```python
from build123d import *

# Parameters (mm, degrees)
SKETCH1_R           = 7.14375
BOSS_EXTRUDE1_DEPTH = 10.25
SKETCH2_R           = 11.75
BOSS_EXTRUDE2_DEPTH = 25
SKETCH6_R           = 4
CUT_EXTRUDE4_DEPTH  = 20
CUT_EXTRUDE5_START  = -20
CUT_EXTRUDE5_DEPTH  = 20
SKETCH7_R           = 4
CUT_EXTRUDE6_DEPTH  = 30
FILLET1_R           = 2.5
FILLET2_R           = 2.5


with BuildPart() as part:
    # Sketch1 → Boss-Extrude1 (new body)
    with BuildSketch(Plane(origin=(0, 0, 0), x_dir=(1, 0, 0), z_dir=(0, 1, 0))):
        with Locations(Location((0, 0, 0), (0, 0, 270))):
            Circle(SKETCH1_R)
    extrude(amount=BOSS_EXTRUDE1_DEPTH)

    # Sketch2 → Boss-Extrude2 (add)
    with BuildSketch(Plane(origin=(0, 10.25, 0), x_dir=(1, 0, 0), z_dir=(0, 1, 0))):
        with Locations(Location((0, 0, 0), (0, 0, 270))):
            Circle(SKETCH2_R)
    extrude(amount=BOSS_EXTRUDE2_DEPTH)

    # Sketch6 → Cut-Extrude4 (cut)
    with BuildSketch(Plane.XZ):
        with Locations(Location((0, 0, 0), (0, 0, 270))):
            Circle(SKETCH6_R)
    extrude(amount=-CUT_EXTRUDE4_DEPTH, mode=Mode.SUBTRACT)

    # Sketch3 → Cut-Extrude5 (cut)
    with BuildSketch(Plane(origin=(0, 35.25, 0), x_dir=(1, 0, 0), z_dir=(0, 1, 0)).offset(CUT_EXTRUDE5_START)):
        with BuildLine():
            ThreePointArc((6.05, 10.072735478), (0, 11.75), (-6.05, 10.072735478))
            Line((-6.05, 10.072735478), (-6.05, -10.072735478))
            ThreePointArc((-6.05, -10.072735478), (0, -11.75), (6.05, -10.072735478))
            Line((6.05, -10.072735478), (6.05, 10.072735478))
        make_face()
        with BuildLine():
            Line((-10.25, -5.744562647), (-10.25, 5.744562647))
            ThreePointArc((-10.25, 5.744562647), (-11.75, 0), (-10.25, -5.744562647))
        make_face()
        with BuildLine():
            ThreePointArc((11.75, 0), (11.368817001, 2.968585522), (10.25, 5.744562647))
            Line((10.25, 5.744562647), (10.25, -5.744562647))
            ThreePointArc((10.25, -5.744562647), (11.368817001, -2.968585522), (11.75, 0))
        make_face()
    extrude(amount=CUT_EXTRUDE5_DEPTH, mode=Mode.SUBTRACT)

    # Sketch7 → Cut-Extrude6 (cut)
    with BuildSketch(Plane.ZY.offset(10.25)):
        with Locations((0, 26.25)):
            Circle(SKETCH7_R)
    extrude(amount=-CUT_EXTRUDE6_DEPTH, mode=Mode.SUBTRACT)

    # Fillet1
    fillet1_edges = [part.edges().sort_by_distance(p)[0] for p in [
        (10.25, 25.25, -5.744562647),
        (10.25, 25.25, 5.744562647),
        (-10.25, 25.25, -5.744562647),
        (-10.25, 25.25, 5.744562647),
    ]]
    fillet(fillet1_edges, radius=FILLET1_R)

    # Fillet2
    fillet2_edges = [part.edges().sort_by_distance(p)[0] for p in [
        (-8.155066755, 35.25, -8.4591599),
        (8.155066755, 35.25, 8.4591599),
        (8.155066755, 35.25, -8.4591599),
        (-8.155066755, 35.25, 8.4591599),
        (10.25, 35.25, 0),
        (10.146506466, 35.25, -5.761620966),
        (10.146506466, 35.25, 5.761620966),
        (-10.25, 35.25, 0),
        (-10.146506466, 35.25, -5.761620966),
        (-10.146506466, 35.25, 5.761620966),
    ]]
    fillet(fillet2_edges, radius=FILLET2_R)


solid = part.part
```
Can you work these out from the model? Positions are in its coordinate system, mm. A direction names the side the tool comes from. Coordinates: 2 decimals unless noted, no trailing zeros. Write each loop counter-clockwise with the first axis right and the second up, starting at its lowest first coordinate (ties: lowest second). Pieces come first, ordered by that corner, then holes. Notation, with made-up numbers: M 3,-36 L 62,-36 A29 cw 62,-13 Z; hole C 30.25,23.5 d4. An arc over 180 degrees is marked long. Write item = value, one per line. Start each with the question number.
Q1. If we section it at D-D, the plane y = 20.5: Write out the boundary of the cut face in (x, z), then the cut area to 3 significant figures.
Q2. If we section it at C-C, the plane z = 0: State how many separate pieces and enclosed holes the cut face has, then the cut area to 3 significant figures.
Q3. I'm going to push flat-ended pins straight in: pin 1 (1 mm diameter, centred on x = 10.5, z = 0, fed in from +Y); pin 2 (5 mm diameter, centred on y = 20.5, z = 0, fed in from -X); pin 3 (10 mm diameter, centred on y = 30, z = 3.5, fed in from +X). Where does each tip first touch, or does it pass through?
Q4. Thinking about a two-plate mould opening in Y: for faces 6 (the face through (-8.179, 30.216, -0.521)), 7 (the face through (11, 15.25, 0)), 8 (the face through (-8, 10.25, 0)), 9 (the face through (8.121, 30.216, -0.521)), which applies, released by +Y, released by -Y, zero draft, split by the parting line, or undercut?
Q5. If we section it at A-A, the plane y = 26.25: Write out the boundary of the cut face in (x, z).
Q6. If I drill on L1, parallel to X at y = 18, z = -3.75; L2, parallel to Y at x = 7.95, z = 0; L3, parallel to Z at x = 0.25, y = 3.5, over which ranges is the centre line in solid material (lowest first)? Write a range as [from, to].
Q7. If we section it at B-B, the plane x = 0: Write out the boundary of the cut face in (y, z).
Q8. On a 3-axis mill with a long thin cutter (end or side, diameter ignored), from which of +Z, -Z, +X, -X, +Y, -Y can I reach the whole of each face in a straight line? I mean faces 1 (the face through (6.05, 21, 0)), 2 (the face through (0.314, 5.053, -7.137)), 3 (the face through (-10.144, 24.123, -5.771)), 4 (the face through (10.144, 24.123, 5.771)), 5 (the face through (-10.25, 22, 0)). Say none if no direction works.
Check sheet entries:
q1.outline = M -10.25,-5.05 A2.5 ccw -9.84,-6.41 A11.75 ccw -6.05,-10.07 L -6.05,10.07 A11.75 ccw -9.84,6.41 A2.5 ccw -10.25,5.05 Z; M 6.05,-10.07 A11.75 ccw 9.84,-6.41 A2.5 ccw 10.25,-5.05 L 10.25,5.05 A2.5 ccw 9.84,6.41 A11.75 ccw 6.05,10.07 Z
q1.area = 139 mm²
q2.separate_pieces = 4
q2.enclosed_holes = 0
q2.area = 240 mm²
q3.pin_1 = 33.84
q3.pin_2 = -10.25
q3.pin_3 = 10.25
q4.face_6 = undercut
q4.face_7 = released by +Y
q4.face_8 = released by -Y
q4.face_9 = undercut
q5.outline = M -10.25,-5.05 A2.5 ccw -9.84,-6.41 A11.75 ccw -6.05,-10.07 L -6.05,-4 L -10.25,-4 Z; M -10.25,4 L -6.05,4 L -6.05,10.07 A11.75 ccw -9.84,6.41 A2.5 ccw -10.25,5.05 Z; M 6.05,-10.07 A11.75 ccw 9.84,-6.41 A2.5 ccw 10.25,-5.05 L 10.25,-4 L 6.05,-4 Z; M 6.05,4 L 10.25,4 L 10.25,5.05 A2.5 ccw 9.84,6.41 A11.75 ccw 6.05,10.07 Z
q6.L1 = [-10.25, -6.05], [6.05, 10.25]
q6.L2 = [10.25, 22.25], [30.25, 35.24]
q6.L3 = [-7.14, -3.99], [3.99, 7.14]
q7.outline = M 0,-7.14 L 10.25,-7.14 L 10.25,-11.75 L 15.25,-11.75 L 15.25,-4 L 0,-4 Z; M 0,4 L 15.25,4 L 15.25,11.75 L 10.25,11.75 L 10.25,7.14 L 0,7.14 Z
q8.face_1 = +Z, -Z, +Y
q8.face_2 = -Y
q8.face_3 = -Z, -X, +Y
q8.face_4 = +Z, +X, +Y
q8.face_5 = +Z, -Z, -X, +Y
